```python
from build123d import *

# Parameters (mm, degrees)
SKETCH_1_R      = 1.7
EXTRUDE_1_DEPTH = 5


with BuildPart() as part:
    # Эскиз1 → Бобышка-Вытянуть1 (new body)
    with BuildSketch(Plane.ZY.offset(-0.758160047)):
        with BuildLine():
            Line((-40.531827395, 59.814835282), (-5.531827395, 59.814835282))
            ThreePointArc((-5.531827395, 59.814835282), (1.93227422, 57.814835282), (-5.531827395, 55.814835282))
            Line((-5.531827395, 55.814835282), (-40.531827395, 55.814835282))
            ThreePointArc((-40.531827395, 55.814835282), (-48.114294617, 57.814835282), (-40.531827395, 59.814835282))
        make_face()
        with Locations((-2.06772578, 57.814835282)):
            Circle(SKETCH_1_R, mode=Mode.SUBTRACT)
        with Locations((-44.059294617, 57.814835282)):
            Circle(SKETCH_1_R, mode=Mode.SUBTRACT)
    extrude(amount=EXTRUDE_1_DEPTH)


solid = part.part
```
Can you work these out from the model? Positions are in its coordinate system, mm. A direction names the side the tool comes from. Round coordinates to 2 decimals unless told otherwise and drop trailing zeros. Order: outer loops, then holes, each group sorted by start corner. A loop starts at its lowest first (then second) coordinate and runs counter-clockwise, first axis right, second up.
(1) If I drill on L1, parallel to Z at x = -3.35, y = 58; L2, parallel to Z at x = -0.3, y = 56.5; L3, parallel to Y at x = -2.95, z = -2, over which ranges is the centre line in solid material (lowest first)?
Results are:
L1: z = -48.11 to -45.75, -42.37 to -3.76, -0.38 to 1.93
L2: z = -47.9 to -45.14, -42.98 to -3.15, -0.99 to 1.71
L3: y = 53.82 to 56.12, 59.51 to 61.81
(2) If we section it at C-C (x = -2.65): Please give me the cut outline in (y, z) (3 decimals), plus the area to 3 significant figures.
Results are:
outline: (55.815, -40.532) arc R4.055 ccw (long way) to (59.815, -40.532) - (59.815, -5.532) arc R4 ccw (long way) to (55.815, -5.532) - close; hole circle Ø3.4 at (57.815, -44.059); hole circle Ø3.4 at (57.815, -2.068)
area: 221 mm2
(3) If we section it at A-A (y = 55): Please give me the cut outline in (x, z), plus the area to 3 significant figures.
Results are:
outline: (-4.24, -46.98) - (0.76, -46.98) - (0.76, -41.14) - (-4.24, -41.14) - close; (-4.24, -4.91) - (0.76, -4.91) - (0.76, 0.77) - (-4.24, 0.77) - close
area: 57.6 mm2
(4) We'd pull the mould along Y, two halves only. Please class faces 3 (the face through (-1.707, 58.964, -3.321)), 4 (the face through (-1.71, 57.96, 1.93)), 5 (the face through (-2, 55.815, -23)), 6 (the face through (-1.707, 57.89, -45.758)): +Y half, -Y half, draft (parallel to the pull), parting line (faces both ways), or undercut.
Results are:
face 3: undercut
face 4: parting line
face 5: -Y half
face 6: undercut
(5) I'm going to push a flat-ended pin straight in: pin 1 (3 mm diameter, centred on x = -1, z = -41, fed in from +Y). Where does the tip first touch, or does it pass through?
Results are:
pin 1: stops at y = 61.56
(6) On a 3-axis mill with a long thin cutter (end or side, diameter ignored), from which of +Z, -Z, +X, -X, +Y, -Y can I reach the whole of each face in a straight line? I mean faces 1 (the face through (-2, 59.815, -23)), 2 (the face through (0.758, 58, -23)). Say none if no direction works.
Results are:
face 1: +X, -X, +Y
face 2: +Z, -Z, +X, +Y, -Y
(7) If we section it at D-D (z = -39): Please give me the cut outline in (x, y), plus the area to 3 significant figures.
Results are:
outline: (-4.24, 55.81) - (0.76, 55.81) - (0.76, 59.81) - (-4.24, 59.81) - close
area: 20.0 mm2
(8) If we section it at B-B (y = 58.75): Please give me the cut outline in (x, z).
Results are:
outline: (-4.24, -48) - (0.76, -48) - (0.76, -45.48) - (-4.24, -45.48) - close; (-4.24, -42.64) - (0.76, -42.64) - (0.76, -3.49) - (-4.24, -3.49) - close; (-4.24, -0.65) - (0.76, -0.65) - (0.76, 1.82) - (-4.24, 1.82) - close
